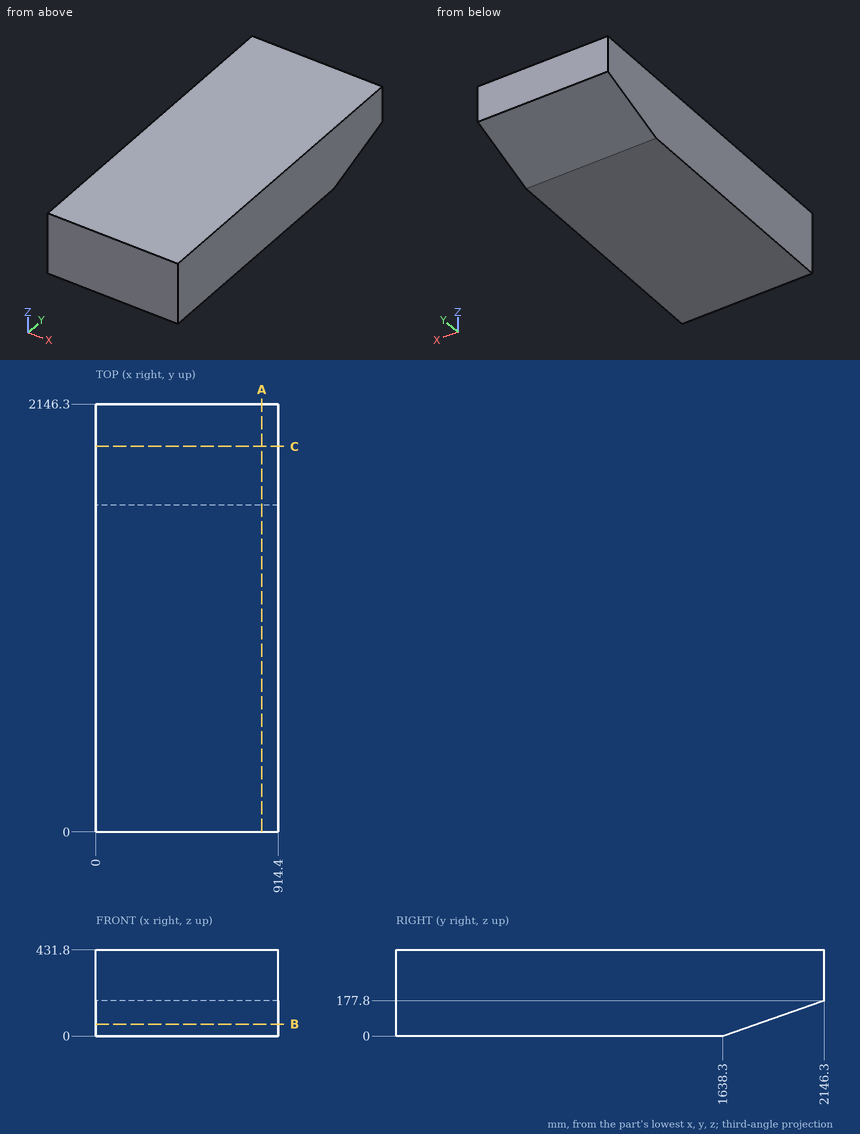
Here's the drawing with two shaded views (mm, measured from the low corner). I have some questions. Coordinates: 2 decimals unless noted, no trailing zeros. Order: outer loops, then holes, each group sorted by start corner. A loop starts at its lowest first (then second) coordinate and runs counter-clockwise, first axis right, second up. Notation, with made-up numbers: (-37, 76) - (-30, 76) arc R9 cw to (-30, 86) - close; hole circle Ø7 at (9, 9). An arc over 180 degrees is marked (long way). Answer in a Markdown table with one row per item.
1. Suppose I cut it at C-C (y = 1934). Please give me the cut outline in (x, z) (3 decimals), and give its area (3 significant figures).
Reply:
| item | result |
|---|---|
| outline | (0, 103.495) - (914.4, 103.495) - (914.4, 431.8) - (0, 431.8) - close |
| area | 300,000 mm^2 |
2. Suppose I cut it at A-A (x = 832). Please give me the cut outline in (y, z).
Reply:
| item | result |
|---|---|
| outline | (0, 0) - (1638.3, 0) - (2146.3, 177.8) - (2146.3, 431.8) - (0, 431.8) - close |
3. For pin 1 (6 mm diameter, centred on y = 533, z = 212.5, fed in from -X), with a flat end and sliding along its axis, tell me the tip position at first contact or that it passes through.
Reply:
| item | result |
|---|---|
| pin 1 | stops at x = 0 |
4. If I drill on line 1 along Z through (x, y) = (138, 1655.5); line 2 along Z through (x, y) = (61.5, 1970.5), over which ranges is the centre line in solid material (lowest first)?
Reply:
| item | result |
|---|---|
| line 1 | z = 6.02 to 431.8 |
| line 2 | z = 116.27 to 431.8 |
5. Suppose I cut it at B-B (z = 59.5). Please give me the cut outline in (x, y), and give its area (3 significant figures).
Reply:
| item | result |
|---|---|
| outline | (0, 0) - (914.4, 0) - (914.4, 1808.3) - (0, 1808.3) - close |
| area | 1,650,000 mm^2 |
